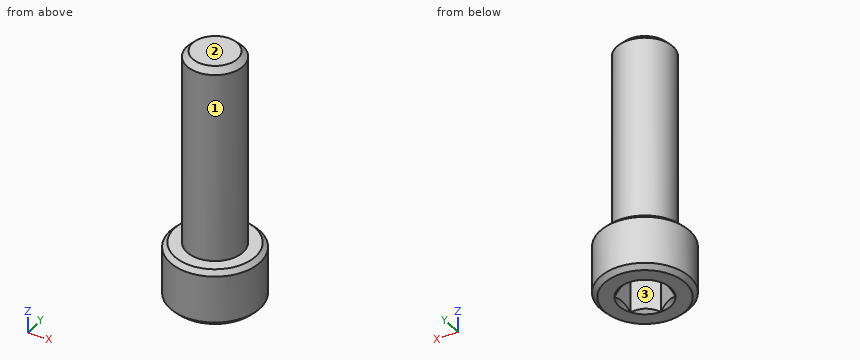
from build123d import *

# Parameters (mm, degrees)
SKETCH1_R          = 5
EXTRUDE1_DEPTH     = 35
SKETCH6_R          = 8
EXTRUDE2_DEPTH     = 10
CUT_EXTRUDE1_DEPTH = 6
CHAMFER1_SIZE      = 0.8
CHAMFER2_SIZE      = 1


with BuildPart() as part:
    # Sketch1 → Extrude1 (new body)
    with BuildSketch(Plane.XY):
        Circle(SKETCH1_R)
    extrude(amount=-EXTRUDE1_DEPTH)

    # Sketch6 → Extrude2 (add)
    with BuildSketch(Plane(origin=(0, 0, -35), x_dir=(-1, 0, 0), z_dir=(0, 0, -1))):
        Circle(SKETCH6_R)
    extrude(amount=EXTRUDE2_DEPTH)

    # Sketch7 → Cut-Extrude1 (cut)
    with BuildSketch(Plane(origin=(0, 0, -45), x_dir=(-1, 0, 0), z_dir=(0, 0, -1))):
        Polygon((0, 4.618802154), (-4, 2.309401077), (-4, -2.309401077), (0, -4.618802154), (4, -2.309401077), (4, 2.309401077), align=None)
    extrude(amount=-CUT_EXTRUDE1_DEPTH, mode=Mode.SUBTRACT)

    # Cut-Extrude2 cone 1 section (through the dimple's axis) → Cut-Extrude2 (revolve, cut)
    with BuildSketch(Plane(origin=(0, 0, -45), x_dir=(0, 1, 0), z_dir=(1, 0, 0))):
        Polygon((0, 0), (4.618802154, 0), (0, 4.618802154), align=None)
    revolve(axis=Axis((0, 0, -45), (0, 0, 1)), mode=Mode.SUBTRACT)

    # Chamfer1
    chamfer1_edges = [part.edges().sort_by_distance(p)[0] for p in [
        (8, 0, -35),
        (8, 0, -45),
    ]]
    chamfer(chamfer1_edges, length=CHAMFER1_SIZE)

    # Chamfer2
    chamfer2_edges = [part.edges().sort_by_distance(p)[0] for p in [
        (-5, 0, 0),
    ]]
    chamfer(chamfer2_edges, length=CHAMFER2_SIZE)


solid = part.part
Design review of the part built by this model. Coordinates are the model's own, in mm. Face numbers are marked on the shaded views. Round coordinates to 2 decimals unless told otherwise and drop trailing zeros. Order: outer loops, then holes, each group sorted by start corner. A loop starts at its lowest first (then second) coordinate and runs counter-clockwise, first axis right, second up. Notation, with made-up numbers: M 48,10 L 102,10 A26 ccw 102,27 Z; hole C -26.75,60.5 d8. An arc over 180 degrees is marked long. Answer as CSV lines item,"result". Start each with the question number.
1) Add section B-B (z = -41). Give the boundary of the cut face in (x, y).
2) The part is to be moulded in two halves that separate along Y. For the marked faces 1, 2 and 3, say which applies: +Y half, -Y half, draft (parallel to the pull), parting line (faces both ways), or undercut.
3) Add section C-C (z = -18). Give the boundary of the cut face in (x, y), then the cut area to 3 significant figures.
4) Add section A-A (y = 0). Give the boundary of the cut face in (x, z), then the cut area to 3 significant figures.
5) Wall thickness on line 1 along Z through (x, y) = (-3, 6); line 2 along Y through (x, z) = (0, -18); line 3 along Z through (x, y) = (2.75, -1): over which ranges is each line inside the solid? List them lowest first. Write a range as [from, to].
6) For pin 1 Ø1.5 at (x, z) = (3, -22.5) entering from -Y; pin 2 Ø6 at (y, z) = (-6.5, -26) entering from -X; pin 3 Ø3 at (y, z) = (-2.5, -20.5) entering from +X, all flat-tipped, find the tip position at first contact; note any pin that passes through.
Resolved:
1,outline,"C 0,0 d16; hole M -4,-2.31 L 0,-4.62 L 4,-2.31 L 4,2.31 L 0,4.62 L -4,2.31 Z"
2,face 1,"parting line"
2,face 2,"draft"
2,face 3,"undercut"
3,outline,"C 0,0 d10"
3,area,"78.5 mm^2"
4,outline,"M -8,-44.2 L -7.2,-45 L -4.62,-45 L -4,-44.38 L -4,-39 L 4,-39 L 4,-44.38 L 4.62,-45 L 7.2,-45 L 8,-44.2 L 8,-35.8 L 7.2,-35 L 5,-35 L 5,-1 L 4,0 L -4,0 L -5,-1 L -5,-35 L -7.2,-35 L -8,-35.8 Z"
4,area,"459 mm^2"
5,line 1,"[-45, -35]"
5,line 2,"[-5, 5]"
5,line 3,"[-39, 0]"
6,pin 1,"y = -4.47"
6,pin 2,"x = -3.57"
6,pin 3,"x = 4.9"
